Read the model definition and answer for the solid it produces. Units are mm, in the model's axes. Give positions to 0.01 mm unless a question says otherwise; leave off trailing zeros. Loops run counter-clockwise (first coordinate to the right, second up) from the corner with the lowest first, then second, coordinate; pieces in that order, holes last. Notation, with made-up numbers: (40, -8.5) -> (88, -8.5) arc R17 ccw to (88, 23.5) -> close; hole circle Ø4 at (4, 46.5). An arc over 180 degrees is marked (long way). Answer as CSV lines item,"result". Start each with the question number.
```python
from build123d import *

# Parameters (mm, degrees)
SKETCH2_W           = 20
SKETCH2_H           = 6
BOSS_EXTRUDE2_DEPTH = 2
CUT_EXTRUDE1_DEPTH  = 6


with BuildPart() as part:
    # Sketch2 → Boss-Extrude2 (new body)
    with BuildSketch(Plane.XY):
        with BuildLine():
            Line((-20, 0), (-20, 6))
            ThreePointArc((-20, 6), (-23, 3), (-20, 0))
        make_face()
        with Locations((-10, 3)):
            Rectangle(SKETCH2_W, SKETCH2_H)
        with BuildLine():
            Line((0, 0), (0, 6))
            ThreePointArc((0, 6), (3, 3), (0, 0))
        make_face()
    extrude(amount=BOSS_EXTRUDE2_DEPTH)

    # Sketch4 → Cut-Extrude1 (cut)
    with BuildSketch(Plane.XY.offset(2)):
        with BuildLine():
            ThreePointArc((-18, 3), (-18.585786438, 4.414213562), (-20, 5))
            Line((-20, 5), (-20, 1))
            ThreePointArc((-20, 1), (-18.585786438, 1.585786438), (-18, 3))
        make_face()
        with BuildLine():
            Line((-20, 1), (-20, 5))
            ThreePointArc((-20, 5), (-22, 3), (-20, 1))
        make_face()
        with BuildLine():
            ThreePointArc((-8, 3), (-8.585786438, 4.414213562), (-10, 5))
            Line((-10, 5), (-10, 1))
            ThreePointArc((-10, 1), (-8.585786438, 1.585786438), (-8, 3))
        make_face()
        with BuildLine():
            Line((-10, 1), (-10, 5))
            ThreePointArc((-10, 5), (-12, 3), (-10, 1))
        make_face()
        with BuildLine():
            ThreePointArc((2, 3), (1.414213562, 4.414213562), (0, 5))
            Line((0, 5), (0, 1))
            ThreePointArc((0, 1), (1.414213562, 1.585786438), (2, 3))
        make_face()
        with BuildLine():
            Line((0, 1), (0, 5))
            ThreePointArc((0, 5), (-2, 3), (0, 1))
        make_face()
    extrude(amount=-CUT_EXTRUDE1_DEPTH, mode=Mode.SUBTRACT)


solid = part.part
```
(1) Find section A-A on z = 1.45. Write down the section's boundary in (x, y).
(2) Find the intervals of material crossed by line 1 along X through (y, z) = (3.7, 1.1); line 2 along X through (y, z) = (4.6, 0.4); line 3 along Y through (x, z) = (-1.5, 1.45), in increasing order. Write a range as from..to.
(3) Find section B-B on x = -1.25. Write down the section's boundary in (y, z), then the cut area to 4 significant figures.
Answer block:
1,outline,"(-20, 0) -> (0, 0) arc R3 ccw to (0, 6) -> (-20, 6) arc R3 ccw to start; hole circle Ø4 at (-20, 3); hole circle Ø4 at (-10, 3); hole circle Ø4 at (0, 3)"
2,line 1,"x = -22.92..-21.87, -18.13..-11.87, -8.13..-1.87, 1.87..2.92"
2,line 2,"x = -22.54..-21.2, -18.8..-11.2, -8.8..-1.2, 1.2..2.54"
2,line 3,"y = 0..1.68, 4.32..6"
3,outline,"(0, 0) -> (1.44, 0) -> (1.44, 2) -> (0, 2) -> close; (4.56, 0) -> (6, 0) -> (6, 2) -> (4.56, 2) -> close"
3,area,"5.755 mm2"
